Check sheet for the modelled part. Datum: model origin and axes. Units: mm. Coordinates: 2 decimals unless noted, no trailing zeros. Write each loop counter-clockwise with the first axis right and the second up, starting at its lowest first coordinate (ties: lowest second). Pieces come first, ordered by that corner, then holes. Notation, with made-up numbers: (-32, 40.25) -> (-23, 40.25) arc R25 ccw to (-23, 61.25) -> close; hole circle Ø9 at (67, -4.75). An arc over 180 degrees is marked (long way). One line per item, written item: value. Start each with the question number.
1) Sectioned sample at C-C on z = 2.75. Enter the section's corners in (x, y), plus the area to 3 significant figures.
2) Scan lines: line 1 along X through (y, z) = (0, 0); line 2 along X through (y, z) = (0, -2.5); line 3 along X through (y, z) = (-4.5, -4.5). Record each from-to range of solid material in increasing order. Write a range as [from, to].
3) Sectioned sample at D-D on y = -4. Enter the section's corners in (x, z) (3 decimals), plus the area to 3 significant figures.
4) Gauge pin test, flat ends, axial feed: P1, Ø3, axis at x = -32.25, y = 0, coming from the -Z side; P2, Ø1, axis at x = 7.5, z = 2, coming from the +Y side. Record the tip position at first contact, or that the pin passes through.
5) Sectioned sample at B-B on x = 22.25. Enter the section's corners in (y, z), plus the area to 3 significant figures.
6) Draft check along X on faces 1 (the flat face through (37.5, 0, 0)), 2 (the flat face through (-1, 6.35, 6)), 3 (the cylindrical face through (9, 0, 0)), 4 (the cylindrical face through (23.47, -0.27, -0.08)). Enter one of: +X half, -X half, draft (parallel to the pull), parting line (faces both ways), or undercut.
7) Sectioned sample at A-A on z = 0. Enter the section's corners in (x, y), plus the area to 3 significant figures.
```python
from build123d import *

# Parameters (mm, degrees)
SKETCH1_W                  = 75
SKETCH1_H                  = 12.7
BOSS_EXTRUDE1_DEPTH        = 6.35
M3_TAPPED_HOLE1_AT_2_COUNT = 2
M3_TAPPED_HOLE1_AT_2_PITCH = 10
M3_TAPPED_HOLE1_AT_3_COUNT = 2
M3_TAPPED_HOLE1_AT_3_PITCH = 54.5
M3_TAPPED_HOLE1_AT_4_COUNT = 2
M3_TAPPED_HOLE1_AT_4_PITCH = 64.5


with BuildPart() as part:
    # Sketch1 → Boss-Extrude1 (new, symmetric)
    with BuildSketch(Plane(origin=(0, 0, 0), x_dir=(1, 0, 0), z_dir=(0, 1, 0))):
        Rectangle(SKETCH1_W, SKETCH1_H)
        with BuildLine():
            ThreePointArc((0, -4.39886349), (-9, 0), (0, 4.39886349))
            ThreePointArc((0, 4.39886349), (5.873085987, 5.008742357), (9, 0))
            ThreePointArc((9, 0), (5.873085987, -5.008742357), (0, -4.39886349))
        make_face(mode=Mode.SUBTRACT)
    extrude(amount=BOSS_EXTRUDE1_DEPTH, both=True)

    # Sketch5 → M3 Tapped Hole1 (revolve, cut)
    with BuildSketch(Plane(origin=(-32.25, 0, -6.35), x_dir=(0, 1, 0), z_dir=(1, 0, 0))):
        Polygon((0, 0), (0, 12.7), (1.75, 12.7), (1.25, 12.2), (1.25, 0.5), (1.75, 0), align=None)
    m3_tapped_hole1 = revolve(axis=Axis((-32.25, 0, -12.7), (0, 0, 1)), mode=Mode.SUBTRACT)

    # M3 Tapped Hole1 at 2: M3 Tapped Hole1 ×2
    with Locations(*[(i * M3_TAPPED_HOLE1_AT_2_PITCH, 0, 0) for i in range(1, M3_TAPPED_HOLE1_AT_2_COUNT)]):
        add(m3_tapped_hole1, mode=Mode.SUBTRACT)

    # M3 Tapped Hole1 at 3: M3 Tapped Hole1 ×2
    with Locations(*[(i * M3_TAPPED_HOLE1_AT_3_PITCH, 0, 0) for i in range(1, M3_TAPPED_HOLE1_AT_3_COUNT)]):
        add(m3_tapped_hole1, mode=Mode.SUBTRACT)

    # M3 Tapped Hole1 at 4: M3 Tapped Hole1 ×2
    with Locations(*[(i * M3_TAPPED_HOLE1_AT_4_PITCH, 0, 0) for i in range(1, M3_TAPPED_HOLE1_AT_4_COUNT)]):
        add(m3_tapped_hole1, mode=Mode.SUBTRACT)


solid = part.part
```
Answers:
1. outline: (-37.5, -6.35) -> (-8.27, -6.35) -> (-8.27, 6.35) -> (-37.5, 6.35) -> close; (8.27, -6.35) -> (37.5, -6.35) -> (37.5, 6.35) -> (8.27, 6.35) -> close; hole circle Ø2.5 at (-32.25, 0); hole circle Ø2.5 at (-22.25, 0); hole circle Ø2.5 at (22.25, 0); hole circle Ø2.5 at (32.25, 0)
1. area: 723 mm2
2. line 1: x = [-37.5, -33.5], [-31, -23.5], [-21, -9], [9, 21], [23.5, 31], [33.5, 37.5]
2. line 2: x = [-37.5, -33.5], [-31, -23.5], [-21, -8.41], [8.41, 21], [23.5, 31], [33.5, 37.5]
2. line 3: x = [-37.5, -6.72], [-0.13, 0.13], [6.72, 37.5]
3. outline: (-37.5, -6.35) -> (37.5, -6.35) -> (37.5, 6.35) -> (-37.5, 6.35) -> close; hole (0, -4.399) arc R5.575 ccw (long way) to (0, 4.399) arc R5.575 ccw (long way) to start
3. area: 784 mm2
4. P1: stops at z = -6.1
4. P2: passes through
5. outline: (-6.35, -6.35) -> (-1.75, -6.35) -> (-1.25, -5.85) -> (-1.25, 5.85) -> (-1.75, 6.35) -> (-6.35, 6.35) -> close; (1.25, -5.85) -> (1.75, -6.35) -> (6.35, -6.35) -> (6.35, 6.35) -> (1.75, 6.35) -> (1.25, 5.85) -> close
5. area: 129 mm2
6. face 1: +X half
6. face 2: draft
6. face 3: undercut
6. face 4: undercut
7. outline: (-37.5, -6.35) -> (-9, -6.35) -> (-9, 6.35) -> (-37.5, 6.35) -> close; (9, -6.35) -> (37.5, -6.35) -> (37.5, 6.35) -> (9, 6.35) -> close; hole circle Ø2.5 at (-32.25, 0); hole circle Ø2.5 at (-22.25, 0); hole circle Ø2.5 at (22.25, 0); hole circle Ø2.5 at (32.25, 0)
7. area: 704 mm2
